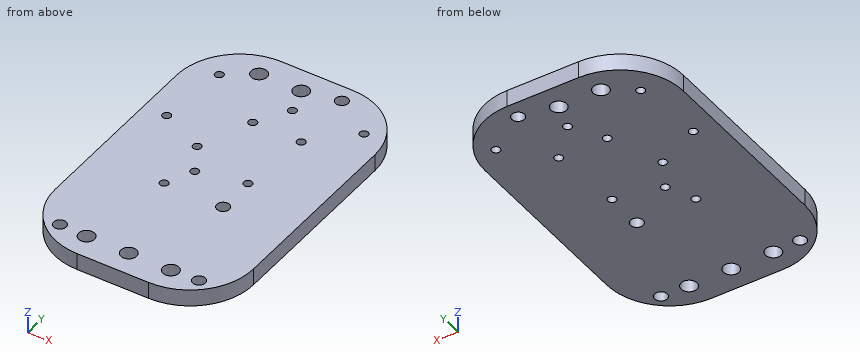
from build123d import *

# Parameters (mm, degrees)
BOARD_DEPTH            = 0.8
SKETCH2_R              = 0.3
SKETCH2_R_2            = 0.375
NON_PLATED_HOLES_DEPTH = 18.79719079
SKETCH3_R              = 0.2
SKETCH3_R_2            = 0.3
PLATED_HOLES_DEPTH     = 18.79719079


with BuildPart() as part:
    # Sketch1 → BOARD (new body)
    with BuildSketch(Plane.XY):
        with BuildLine():
            Line((0.3, 11.9), (0.3, 3.1))
            ThreePointArc((0.3, 3.1), (1.178679656, 0.978679656), (3.3, 0.1))
            Line((3.3, 0.1), (6.7, 0.1))
            ThreePointArc((6.7, 0.1), (8.821320344, 0.978679656), (9.7, 3.1))
            Line((9.7, 3.1), (9.7, 11.9))
            ThreePointArc((9.7, 11.9), (8.821320344, 14.021320344), (6.7, 14.9))
            Line((6.7, 14.9), (3.3, 14.9))
            ThreePointArc((3.3, 14.9), (1.178679656, 14.021320344), (0.3, 11.9))
        make_face()
    extrude(amount=BOARD_DEPTH)

    # Sketch2 → NON-PLATED HOLES (cut, through all)
    with BuildSketch(Plane.XY):
        with Locations((1.7, 1.3)):
            Circle(SKETCH2_R)
        with Locations((8.3, 1.3)):
            Circle(SKETCH2_R)
        with Locations((6.7, 14.1)):
            Circle(SKETCH2_R)
        with Locations((5, 13.75)):
            Circle(SKETCH2_R_2)
        with Locations((3, 13.75)):
            Circle(SKETCH2_R_2)
        with Locations((3, 1.25)):
            Circle(SKETCH2_R_2)
        with Locations((5, 1.25)):
            Circle(SKETCH2_R_2)
        with Locations((7, 1.25)):
            Circle(SKETCH2_R_2)
    extrude(amount=NON_PLATED_HOLES_DEPTH, mode=Mode.SUBTRACT)

    # Sketch3 → PLATED HOLES (cut, through all)
    with BuildSketch(Plane.XY):
        with Locations((4.5, 11)):
            Circle(SKETCH3_R)
        with Locations((1.4, 9.5)):
            Circle(SKETCH3_R)
        with Locations((8.6, 12.8)):
            Circle(SKETCH3_R)
        with Locations((1.7, 12.85)):
            Circle(SKETCH3_R)
        with Locations((3.5, 8.5)):
            Circle(SKETCH3_R)
        with Locations((3.7, 5.8)):
            Circle(SKETCH3_R)
        with Locations((6.8, 11)):
            Circle(SKETCH3_R)
        with Locations((6.5, 7.6)):
            Circle(SKETCH3_R)
        with Locations((6.5, 5.8)):
            Circle(SKETCH3_R_2)
        with Locations((4.3, 7.1)):
            Circle(SKETCH3_R)
        with Locations((5.4, 12.5)):
            Circle(SKETCH3_R)
    extrude(amount=PLATED_HOLES_DEPTH, mode=Mode.SUBTRACT)


solid = part.part
Read the model definition and answer for the solid it produces. Units are mm, in the model's axes. Give positions to 0.01 mm unless a question says otherwise; leave off trailing zeros. Write each loop counter-clockwise with the first axis right and the second up, starting at its lowest first coordinate (ties: lowest second). Pieces come first, ordered by that corner, then holes. Notation, with made-up numbers: (70.5, 33) - (108.5, 33) arc R11 ccw to (108.5, 51) - close; hole circle Ø3 at (-18, -4.75). An arc over 180 degrees is marked (long way). Use CSV: the item, a comma, the result in double quotes. Start each with the question number.
(1) Find section C-C (x = 3). Give the vertices of the cut face in (y, z) (3 decimals), plus the area to 3 significant figures.
(2) Consider line 1 along Y through (x, z) = (5, 0.55) (3 decimals); line 2 along X through (y, z) = (7.1, 0.65); line 3 along Y through (x, z) = (6.5, 0.3). Determine where each line is inside the solid, lowest interval first.
(3) Find section D-D (x = 1). Give the vertices of the cut face in (y, z), plus the area to 3 significant figures.
(4) Find section A-A (z = 0.15). Count the separate pieces of the cut face and the enclosed holes in it, plus the area to 3 significant figures.
(5) Find section B-B (y = 7.1). Give the vertices of the cut face in (x, z).
Findings below:
1,outline,"(0.115, 0) - (0.875, 0) - (0.875, 0.8) - (0.115, 0.8) - close; (1.625, 0) - (13.375, 0) - (13.375, 0.8) - (1.625, 0.8) - close; (14.125, 0) - (14.885, 0) - (14.885, 0.8) - (14.125, 0.8) - close"
1,area,"10.6 mm2"
2,line 1,"0.1 to 0.875, 1.625 to 13.375, 14.125 to 14.9"
2,line 2,"0.3 to 4.1, 4.5 to 9.7"
2,line 3,"0.1 to 5.5, 6.1 to 7.4, 7.8 to 13.88, 14.32 to 14.9"
3,outline,"(1.17, 0) - (13.83, 0) - (13.83, 0.8) - (1.17, 0.8) - close"
3,area,"10.1 mm2"
4,separate pieces,"1"
4,enclosed holes,"19"
4,area,"127 mm2"
5,outline,"(0.3, 0) - (4.1, 0) - (4.1, 0.8) - (0.3, 0.8) - close; (4.5, 0) - (9.7, 0) - (9.7, 0.8) - (4.5, 0.8) - close"
